```python
from build123d import *

# Parameters (mm, degrees)
SKETCH_1_R          = 7.5
EXTRUDE_2_DEPTH     = 16
SKETCH_2_R          = 3.5
CUT_EXTRUDE_1_DEPTH = 16


with BuildPart() as part:
    # 草图1 → 凸台-拉伸2 (new body)
    with BuildSketch(Plane.XY):
        with BuildLine():
            Line((15.402921801, -15), (21.5, -15))
            Line((21.5, -15), (21.5, 0))
            ThreePointArc((21.5, 0), (19.917490037, -8.095899619), (15.402921801, -15))
        make_face()
        with BuildLine():
            ThreePointArc((21.5, 0), (0, 21.5), (-21.5, 0))
            ThreePointArc((-21.5, 0), (-19.917490037, -8.095899619), (-15.402921801, -15))
            Line((-15.402921801, -15), (15.402921801, -15))
            ThreePointArc((15.402921801, -15), (19.917490037, -8.095899619), (21.5, 0))
        make_face()
        Circle(SKETCH_1_R, mode=Mode.SUBTRACT)
        with BuildLine():
            Line((-21.5, 0), (-21.5, -15))
            Line((-21.5, -15), (-15.402921801, -15))
            ThreePointArc((-15.402921801, -15), (-19.917490037, -8.095899619), (-21.5, 0))
        make_face()
        with BuildLine():
            Line((-40, -22), (0, -22))
            Line((0, -22), (40, -22))
            Line((40, -22), (40.439940075, -22))
            Line((40.439940075, -22), (40.439940075, -15))
            Line((40.439940075, -15), (21.5, -15))
            Line((21.5, -15), (15.402921801, -15))
            ThreePointArc((15.402921801, -15), (0, -21.5), (-15.402921801, -15))
            Line((-15.402921801, -15), (-21.5, -15))
            Line((-21.5, -15), (-40, -15))
            Line((-40, -15), (-40, -22))
        make_face()
        with BuildLine():
            Line((15.402921801, -15), (-15.402921801, -15))
            ThreePointArc((-15.402921801, -15), (0, -21.5), (15.402921801, -15))
        make_face()
    extrude(amount=EXTRUDE_2_DEPTH)

    # 草图2 → 切除-拉伸1 (cut)
    with BuildSketch(Plane(origin=(0, -15, 0), x_dir=(1, 0, 0), z_dir=(0, 1, 0))):
        with Locations((-30.75, -8)):
            Circle(SKETCH_2_R)
        with Locations((30.969970037, -8)):
            Circle(SKETCH_2_R)
    extrude(amount=-CUT_EXTRUDE_1_DEPTH, mode=Mode.SUBTRACT)


solid = part.part
```
For this review, take the finished solid that the model builds, in its own axes (mm). A direction names the side the tool comes from. Round coordinates to 2 decimals unless told otherwise and drop trailing zeros. Loops run counter-clockwise (first coordinate to the right, second up) from the corner with the lowest first, then second, coordinate; pieces in that order, holes last.
Q1. Add section B-B on z = 9.5. Write out the cut boundary in (x, y), plus the area to 3 significant figures.
Result sheet:
outline: (-40, -22) - (-33.91, -22) - (-33.91, -15) - (-40, -15) - close; (-27.59, -22) - (27.81, -22) - (27.81, -15) - (21.5, -15) - (21.5, 0) arc R21.5 ccw to (-21.5, 0) - (-21.5, -15) - (-27.59, -15) - close; (34.13, -22) - (40.44, -22) - (40.44, -15) - (34.13, -15) - close; hole circle Ø15 at (0, 0)
area: 1,670 mm2
Q2. To check wall thickness, follow line 1 along X through (y, z) = (-17.25, 8); line 2 along Y through (x, z) = (0, 4.25); line 3 along Y through (x, z) = (31.5, 4.25). State the ranges of each line that lie inside material, in increasing order.
Result sheet:
line 1: x = -40 to -34.25, -27.25 to 27.47, 34.47 to 40.44
line 2: y = -22 to -7.5, 7.5 to 21.5
line 3: y = -22 to -15
Q3. Add section C-C on y = 1. Write out the cut boundary in (x, z), plus the area to 3 significant figures.
Result sheet:
outline: (-21.48, 0) - (-7.43, 0) - (-7.43, 16) - (-21.48, 16) - close; (7.43, 0) - (21.48, 0) - (21.48, 16) - (7.43, 16) - close
area: 449 mm2
Q4. Mouldability with a two-part tool opening along X and no side actions: class faces 1 (the face through (27.473, -18.451, 7.846)), 2 (the face through (-7.493, 0.33, 7.888)), 3 (the face through (-31, -15, 4)), 4 (the face through (0.473, 21.495, 7.888)) as +X half, -X half, draft (parallel to the pull), parting line (faces both ways), or undercut.
Result sheet:
face 1: undercut
face 2: undercut
face 3: draft
face 4: parting line
Q5. Add section D-D on z = 14.25. Write out the cut boundary in (x, y), plus the area to 3 significant figures.
Result sheet:
outline: (-40, -22) - (40.44, -22) - (40.44, -15) - (21.5, -15) - (21.5, 0) arc R21.5 ccw to (-21.5, 0) - (-21.5, -15) - (-40, -15) - close; hole circle Ø15 at (0, 0)
area: 1,760 mm2
Q6. Insertion check: pin 1 Ø1 at (x, z) = (-14, 6) entering from +Y; pin 2 Ø8 at (x, z) = (-30.75, 8) entering from +Y; pin 3 Ø2 at (x, z) = (3.5, 3) entering from +Y; pin 4 Ø6 at (x, y) = (-5.5, 10.5) entering from -Z. Each pin has a flat end and moves straight along its axis. Give the tip position at first contact, or say it passes through.
Result sheet:
pin 1: stops at y = 16.73
pin 2: stops at y = -15
pin 3: stops at y = 21.35
pin 4: stops at z = 0
Q7. Add section A-A on x = 0. Write out the cut boundary in (y, z).
Result sheet:
outline: (-22, 0) - (-7.5, 0) - (-7.5, 16) - (-22, 16) - close; (7.5, 0) - (21.5, 0) - (21.5, 16) - (7.5, 16) - close
Q8. Machinability: for faces 5 (the face through (-21.5, -7, 8)), 6 (the face through (21.5, -8, 8)), 7 (the face through (0, -22, 8)), which of the approach directions +Z, -Z, +X, -X, +Y, -Y give a long, thin tool a straight path to every point of the face, cutting with its end or side? Answer none if there is none.
Result sheet:
face 5: +Z, -Z, -X, +Y
face 6: +Z, -Z, +X, +Y
face 7: +Z, -Z, +X, -X, -Y
